Design review of the part built by this model. Coordinates are the model's own, in mm. Give positions to 0.01 mm unless a question says otherwise; leave off trailing zeros. Order: outer loops, then holes, each group sorted by start corner. A loop starts at its lowest first (then second) coordinate and runs counter-clockwise, first axis right, second up.
```python
from build123d import *

# Parameters (mm, degrees)
SKETCH_3_R          = 60.3
EXTRUDE_2_DEPTH     = 10
CUT_EXTRUDE_2_DEPTH = 11
FILLET_1_R          = 3
SKETCH_5_R          = 1.25
CUT_EXTRUDE_3_DEPTH = 11
SKETCH_6_R          = 5.1
CUT_EXTRUDE_4_DEPTH = 11
SKETCH_7_R          = 5.1
CUT_EXTRUDE_5_DEPTH = 11


with BuildPart() as part:
    # 草图3 → 凸台-拉伸2 (new body)
    with BuildSketch(Plane(origin=(0, 0, 0), x_dir=(1, 0, 0), z_dir=(0, 1, 0))):
        Circle(SKETCH_3_R)
    extrude(amount=EXTRUDE_2_DEPTH)

    # 草图4 → 切除-拉伸2 (cut, through all)
    with BuildSketch(Plane(origin=(0, 10, 0), x_dir=(1, 0, 0), z_dir=(0, 1, 0))):
        with BuildLine():
            Line((-51.556667852, 20), (-56.886641666, 20))
            ThreePointArc((-56.886641666, 20), (0, 60.3), (56.886641666, 20))
            Line((56.886641666, 20), (51.556667852, 20))
            ThreePointArc((51.556667852, 20), (0, 55.3), (-51.556667852, 20))
        make_face()
        with BuildLine():
            Line((-56.886641666, -20), (-51.556667852, -20))
            ThreePointArc((-51.556667852, -20), (0, -55.3), (51.556667852, -20))
            Line((51.556667852, -20), (56.886641666, -20))
            ThreePointArc((56.886641666, -20), (0, -60.3), (-56.886641666, -20))
        make_face()
    extrude(amount=-CUT_EXTRUDE_2_DEPTH, mode=Mode.SUBTRACT)

    # 圆角1
    fillet_1_edges = [part.edges().sort_by_distance(p)[0] for p in [
        (51.556667852, 5, -20),
        (-51.556667852, 5, -20),
        (-56.886641666, 5, -20),
        (56.886641666, 5, -20),
        (-51.556667852, 5, 20),
        (51.556667852, 5, 20),
        (56.886641666, 5, 20),
        (-56.886641666, 5, 20),
    ]]
    fillet(fillet_1_edges, radius=FILLET_1_R)

    # 草图5 → 切除-拉伸3 (cut, through all)
    with BuildSketch(Plane.XZ):
        with Locations((0, -52.7)):
            Circle(SKETCH_5_R)
        with Locations((-45.639538779, -26.35)):
            Circle(SKETCH_5_R)
        with Locations((-45.639538779, 26.35)):
            Circle(SKETCH_5_R)
        with Locations((0, 52.7)):
            Circle(SKETCH_5_R)
        with Locations((45.639538779, 26.35)):
            Circle(SKETCH_5_R)
        with Locations((45.639538779, -26.35)):
            Circle(SKETCH_5_R)
    extrude(amount=-CUT_EXTRUDE_3_DEPTH, mode=Mode.SUBTRACT)

    # 草图6 → 切除-拉伸4 (cut, through all)
    with BuildSketch(Plane(origin=(0, 10, 0), x_dir=(1, 0, 0), z_dir=(0, 1, 0))):
        with Locations((0, 31)):
            Circle(SKETCH_6_R)
        with Locations((24.236775957, 19.328183858)):
            Circle(SKETCH_6_R)
        with Locations((30.222765278, -6.898148953)):
            Circle(SKETCH_6_R)
        with Locations((13.450395913, -27.930034905)):
            Circle(SKETCH_6_R)
        with Locations((-13.450395913, -27.930034905)):
            Circle(SKETCH_6_R)
        with Locations((-30.222765278, -6.898148953)):
            Circle(SKETCH_6_R)
        with Locations((-24.236775957, 19.328183858)):
            Circle(SKETCH_6_R)
    extrude(amount=-CUT_EXTRUDE_4_DEPTH, mode=Mode.SUBTRACT)

    # 草图7 → 切除-拉伸5 (cut, through all)
    with BuildSketch(Plane(origin=(0, 10, 0), x_dir=(1, 0, 0), z_dir=(0, 1, 0))):
        with Locations((0, 12)):
            Circle(SKETCH_7_R)
        with Locations((10.392304845, -6)):
            Circle(SKETCH_7_R)
        with Locations((-10.392304845, -6)):
            Circle(SKETCH_7_R)
    extrude(amount=-CUT_EXTRUDE_5_DEPTH, mode=Mode.SUBTRACT)


solid = part.part
```
1. For line 1 along X through (y, z) = (4.75, -25.5); line 2 along Z through (x, y) = (11, 6.25); line 3 along Z through (x, y) = (-26.5, 7.75), list the stretches that pass through material, from the lowest coordinate up.
Recorded:
line 1: x = -49.07 to -46.56, -44.72 to 44.72, 46.56 to 49.07
line 2: z = -54.19 to 0.94, 11.06 to 23.46, 32.4 to 54.19
line 3: z = -48.54 to -23.9, -14.76 to 3.41, 10.38 to 48.54
2. For pin 1 (1 mm diameter, centred on y = 2, z = 1, fed in from -X); pin 2 (4 mm diameter, centred on x = -32.5, y = 3, fed in from +Z); pin 3 (2 mm diameter, centred on x = 0, z = 52.7, fed in from +Y); pin 4 (0.6 mm diameter, centred on x = -54.5, y = 3.5, fed in from -Z), all flat-tipped, find the tip position at first contact; note any pin that passes through.
Recorded:
pin 1: stops at x = -60.3
pin 2: stops at z = 46.13
pin 3: passes through
pin 4: stops at z = -20
3. Take a section at D-D (y = 1.75). State how many separate pieces and enclosed holes the cut face has, then the cut area to 3 significant figures.
Recorded:
separate pieces: 1
enclosed holes: 16
area: 9,170 mm2
4. Take a section at A-A (z = -12). State the section outline as (x, y) points, then the cut area to 3 significant figures.
Recorded:
outline: (-59.09, 0) - (-5.1, 0) - (-5.1, 10) - (-59.09, 10) - close; (5.1, 0) - (59.09, 0) - (59.09, 10) - (5.1, 10) - close
area: 1,080 mm2
5. Draft analysis for pull direction Z (two halves, no side actions). For faces 1 (the face through (9.4, 5.07, 31.03)), 2 (the face through (51.9, 4.93, 20.51)), 3 (the face through (-1, 10, -1)), state which applies: pulls with the +Z half, pulls with the -Z half, needs draft (parallel to the pull), parting line crosses it, or undercut.
Recorded:
face 1: undercut
face 2: pulls with the +Z half
face 3: needs draft
6. Take a section at B-B (x = -17). State the section outline as (y, z) points, then the cut area to 3 significant figures.
Recorded:
outline: (0, -52.62) - (10, -52.62) - (10, 24.27) - (0, 24.27) - close; (0, 31.59) - (10, 31.59) - (10, 52.62) - (0, 52.62) - close
area: 979 mm2
7. Take a section at C-C (x = 11). State the section outline as (y, z) points, then the cut area to 3 significant figures.
Recorded:
outline: (0, -54.19) - (10, -54.19) - (10, 0.94) - (0, 0.94) - close; (0, 11.06) - (10, 11.06) - (10, 23.46) - (0, 23.46) - close; (0, 32.4) - (10, 32.4) - (10, 54.19) - (0, 54.19) - close
area: 893 mm2
